Autodesk Inventor part; units mm, degrees
ref_plane "YZ Plane" through (0, 0, 0) normal (1, 0, 0) x (0, 1, 0)
ref_plane "XZ Plane" through (0, 0, 0) normal (0, 1, 0) x (-1, 0, 0)
ref_plane "XY Plane" through (0, 0, 0) normal (0, 0, 1) x (1, 0, 0)
sketch "스케치3" plane through (0, 0, 0) normal (0, 1, 0) x (-1, 0, 0)
  line L0 (34.9919, -14.4941) -> (14.4941, -34.9919)
  line L1 (14.4941, -34.9919) -> (-14.4941, -34.9919)
  line L2 (-14.4941, -34.9919) -> (-34.9919, -14.4941)
  line L3 (-34.9919, -14.4941) -> (-34.9919, 14.4941)
  line L4 (-34.9919, 14.4941) -> (-14.4941, 34.9919)
  line L5 (-14.4941, 34.9919) -> (14.4941, 34.9919)
  line L6 (14.4941, 34.9919) -> (34.9919, 14.4941)
  line L7 (34.9919, 14.4941) -> (34.9919, -14.4941)
  line L8 (13.5, -32.5919) -> (-13.5, -32.5919)
  line L9 (-13.5, -32.5919) -> (-32.5919, -13.5)
  line L10 (-32.5919, -13.5) -> (-32.5919, 13.5)
  line L11 (-32.5919, 13.5) -> (-13.5, 32.5919)
  line L12 (-13.5, 32.5919) -> (13.5, 32.5919)
  line L13 (13.5, 32.5919) -> (32.5919, 13.5)
  line L14 (32.5919, 13.5) -> (32.5919, -13.5)
  line L15 (32.5919, -13.5) -> (13.5, -32.5919)
  point P0 (0, 0)
  point P1 (0, 0)
  point P2 (0, 0)
  point P3 (0, 0)
  dimension "d66" = 27
  dimension "d67" = 2.4
extrude "돌출2" add sketch "스케치3" along normal blind 3.4 contours L0 L1 L2 L3 L4 L5 L6 L7 | L8 L9 L10 L11 L12 L13 L14 L15
sketch "스케치4" plane through (0, 3.4, 0) normal (0, 1, 0) x (1, 0, 0)
  line L0 (13.5, -32.5919) -> (-13.5, -32.5919)
  line L1 (-13.5, -32.5919) -> (-32.5919, -13.5)
  line L2 (-32.5919, -13.5) -> (-32.5919, 13.5)
  line L3 (-32.5919, 13.5) -> (-13.5, 32.5919)
  line L4 (-13.5, 32.5919) -> (13.5, 32.5919)
  line L5 (13.5, 32.5919) -> (32.5919, 13.5)
  line L6 (32.5919, 13.5) -> (32.5919, -13.5)
  line L7 (32.5919, -13.5) -> (13.5, -32.5919)
  line L8 (-13.9971, 33.7919) -> (13.9971, 33.7919)
  line L9 (13.9971, 33.7919) -> (33.7919, 13.9971)
  line L10 (33.7919, 13.9971) -> (33.7919, -13.9971)
  line L11 (33.7919, -13.9971) -> (13.9971, -33.7919)
  line L12 (13.9971, -33.7919) -> (-13.9971, -33.7919)
  line L13 (-13.9971, -33.7919) -> (-33.7919, -13.9971)
  line L14 (-33.7919, -13.9971) -> (-33.7919, 13.9971)
  line L15 (-33.7919, 13.9971) -> (-13.9971, 33.7919)
  line L16 (-13.1686, 31.7919) -> (13.1686, 31.7919)
  line L17 (13.1686, 31.7919) -> (31.7919, 13.1686)
  line L18 (31.7919, 13.1686) -> (31.7919, -13.1686)
  line L19 (31.7919, -13.1686) -> (13.1686, -31.7919)
  line L20 (13.1686, -31.7919) -> (-13.1686, -31.7919)
  line L21 (-13.1686, -31.7919) -> (-31.7919, -13.1686)
  line L22 (-31.7919, -13.1686) -> (-31.7919, 13.1686)
  line L23 (-31.7919, 13.1686) -> (-13.1686, 31.7919)
  point P0 (0, 0)
  point P1 (0, 0)
  point P2 (0, 0)
  point P3 (0, 0)
  dimension "d7" = 27
  dimension "d68" = 1.2
  dimension "d69" = 0.8
extrude "돌출3" cut sketch "스케치4" against normal blind 1.2 contours L0 L1 L2 L3 L4 L5 L6 L7 | L8 L9 L10 L11 L12 L13 L14 L15 | L16 L17 L18 L19 L20 L21 L22 L23
sketch "스케치9" plane through (0, 0, 0) normal (0, -1, 0) x (1, 0, 0)
  line L0 (7.5, 10) -> (2.5, 10)
  line L1 (2.5, 10) -> (2.5, -10)
  line L2 (2.5, -10) -> (7.5, -10)
  line L3 (7.5, -10) -> (7.5, 10)
  line L4 (7.5, 10) -> (2.5, -10) construction
  line L5 (2.5, 10) -> (7.5, -10) construction
  line L6 (-2.5, 10) -> (-7.5, 10)
  line L7 (-7.5, 10) -> (-7.5, -10)
  line L8 (-7.5, -10) -> (-2.5, -10)
  line L9 (-2.5, 10) -> (-7.5, -10) construction
  line L10 (-7.5, 10) -> (-2.5, -10) construction
  line L11 (-2.5, -10) -> (-2.5, 10)
  point P0 (0, 0)
  point P1 (5, 0)
  point P2 (-5, 0)
  dimension "d42" = 20
  dimension "d43" = 5
  dimension "d44" = 2.5
  dimension "d47" = 10
extrude "돌출8" add sketch "스케치9" along normal blind 10
sketch "스케치10" plane through (-7.5, 0, -10) normal (-1, 0, 0) x (0, 0, 1)
  circle A0 centre (15, -5) radius 1.25
  line L0 (19.9591, 0) -> (0.0886, 0)
  line L1 (24.4941, 0) -> (-4.4941, 0)
  circle A1 centre (5, -5) radius 1.25
  line L2 (20, 0) -> (20, -10)
  point P0 (10, 0)
  dimension "d54" = 2.5
  dimension "d57" = 10
  dimension "d62" = 5
  dimension "d63" = 5
extrude "돌출9" cut sketch "스케치10" against normal blind 20
sketch "스케치11" plane through (0, 2.2, 0) normal (0, 1, 0) x (1, 0, 0)
  line L0 (-13.1686, 31.7919) -> (13.1686, 31.7919)
  line L1 (13.1686, 31.7919) -> (31.7919, 13.1686)
  line L2 (31.7919, 13.1686) -> (31.7919, -13.1686)
  line L3 (31.7919, -13.1686) -> (13.1686, -31.7919)
  line L4 (13.1686, -31.7919) -> (-13.1686, -31.7919)
  line L5 (-13.1686, -31.7919) -> (-31.7919, -13.1686)
  line L6 (-31.7919, -13.1686) -> (-31.7919, 13.1686)
  line L7 (-31.7919, 13.1686) -> (-13.1686, 31.7919)
  line L8 (-13.9971, 33.7919) -> (13.9971, 33.7919)
  line L9 (-11.926, 28.7919) -> (11.926, 28.7919)
  line L10 (11.926, 28.7919) -> (28.7919, 11.926)
  line L11 (28.7919, 11.926) -> (28.7919, -11.926)
  line L12 (28.7919, -11.926) -> (11.926, -28.7919)
  line L13 (11.926, -28.7919) -> (-11.926, -28.7919)
  line L14 (-11.926, -28.7919) -> (-28.7919, -11.926)
  line L15 (-28.7919, -11.926) -> (-28.7919, 11.926)
  line L16 (-28.7919, 11.926) -> (-11.926, 28.7919)
  point P0 (0, 0)
  point P1 (0, 0)
  point P2 (0, 0)
  dimension "d70" = 2
  dimension "d71" = 3
extrude "돌출10" add sketch "스케치11" along normal blind 0.6 contours L0 L1 L2 L3 L4 L5 L6 L7 | L9 L10 L11 L12 L13 L14 L15 L16
fillet "모깎기1" radius 1.2 16 edges at (-24.743, 3.4, 24.743) (0, 3.4, 34.9919) (24.743, 3.4, 24.743) (34.9919, 3.4, 0) (24.743, 3.4, -24.743) (0, 3.4, -34.9919) (-24.743, 3.4, -24.743) (-34.9919, 3.4, 0) (-24.743, 0, 24.743) (0, 0, 34.9919) (24.743, 0, 24.743) (34.9919, 0, 0) (24.743, 0, -24.743) (0, 0, -34.9919) (-24.743, 0, -24.743) (-34.9919, 0, 0)
properties part number "OV-PAM_bottom_2"
Input: part model. Units: mm. Frame: model coordinates. A direction names the side the tool comes from. Round coordinates to 2 decimals unless told otherwise and drop trailing zeros. Write each loop counter-clockwise with the first axis right and the second up, starting at its lowest first coordinate (ties: lowest second). Pieces come first, ordered by that corner, then holes. Notation, with made-up numbers: M -23.5,73.5 L 29.5,73.5 A21 cw 29.5,98.5 Z; hole C 50.25,64.25 d8. An arc over 180 degrees is marked long. Write each question's results on one line, items separated by ' | '.
Q1. Section query A-A (y = -7.5). Return loops of the section in (x, z), and give its area (3 significant figures).
Results:
outline: M -7.5,-10 L -2.5,-10 L -2.5,10 L -7.5,10 Z; M 2.5,-10 L 7.5,-10 L 7.5,10 L 2.5,10 Z | area: 200 mm^2
Q2. Line query: line 1 along Y through (x, z) = (6, 5); line 2 along X through (y, z) = (2.25, 4.5); line 3 along Y through (x, z) = (-12, 7). Output: solid intervals per line, ascending.
Results:
line 1: y = -10 to -6.25, -3.75 to 2.8 | line 2: x = -34.99 to -33.79, -31.79 to 31.79, 33.79 to 34.99 | line 3: y = 0 to 2.8
Q3. Draft query along X for faces 1 (the face through (5, -5, 10)), 2 (the face through (-24.36, 3.04, -24.64)), 3 (the face through (2.5, -5, 0)). Return one class per face: released by +X, released by -X, zero draft, split by the parting line, or undercut.
Results:
face 1: zero draft | face 2: released by -X | face 3: undercut
Q4. Section query B-B (z = -5). State how many separate pieces and enclosed holes the cut face has, and give its area (3 significant figures).
Results:
separate pieces: 3 | enclosed holes: 0 | area: 269 mm^2
Q5. Access query for faces 4 (the face through (-7.5, -5, 0)), 5 (the face through (-24.6, 1.693, 24.886)), 6 (the face through (-2.5, -5, 0)), 7 (the face through (-24.03, 2.81, -23.76)). Directions: +Z, -Z, +X, -X, +Y, -Y. A direction counts if a zero-diameter tool reaches every point of the face in a straight line with its end or side. Return the directions, or none.
Results:
face 4: +Z, -Z, -X, -Y | face 5: +Z, -X, +Y, -Y | face 6: +Z, -Z, -Y | face 7: +Y
Q6. Pin query (flat end, axial travel): P1, Ø1, axis at y = -7.5, z = 3.5, coming from the +X side; P2, Ø0.7, axis at x = -6, y = 2.5, coming from the -Z side; P3, Ø6, axis at x = -27, y = -5, coming from the -Z side; P4, Ø1, axis at x = -3, z = -23, coming from the -Y side. Return the tip coordinate at first contact, or that it passes through.
Results:
P1: stops at x = 7.5 | P2: stops at z = -34.99 | P3: passes through | P4: stops at y = 0
